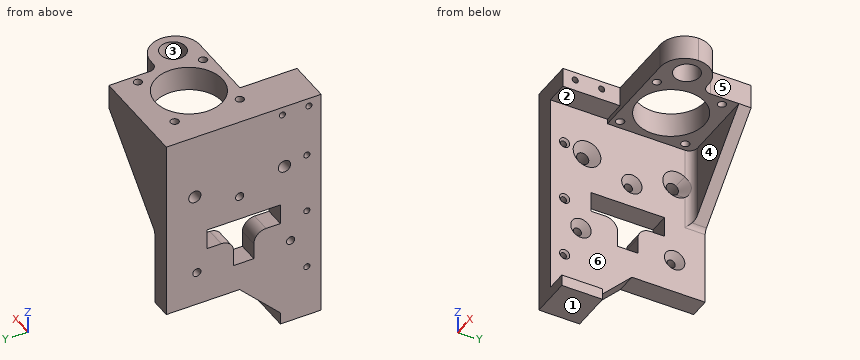
Autodesk Inventor part; units mm, degrees
ref_plane "YZ Plane" through (0, 0, 0) normal (1, 0, 0) x (0, 1, 0)
ref_plane "XZ Plane" through (0, 0, 0) normal (0, 1, 0) x (-1, 0, 0)
ref_plane "XY Plane" through (0, 0, 0) normal (0, 0, 1) x (1, 0, 0)
sketch "Sketch1" plane through (0, 0, 0) normal (1, 0, 0) x (0, 1, 0)
  line L0 (-23.3447, 18.3788) -> (14.6553, 18.3788)
  line L1 (14.6553, 18.3788) -> (14.6553, -36.6212)
  line L2 (14.6553, -36.6212) -> (-23.3447, -36.6212)
  line L3 (-23.3447, -36.6212) -> (-23.3447, 18.3788)
  point P0 (0, 0)
  dimension "d0" = 38
  dimension "d1" = 55
extrude "Extrusion1" add sketch "Sketch1" along normal blind 5
sketch "Sketch2" plane through (5, 0, 0) normal (1, 0, 0) x (0, 0, -1)
  line L0 (36.6212, 14.6553) -> (-18.3788, 14.6553)
  line L1 (-18.3788, 14.6553) -> (-12.3788, 14.6553)
  line L2 (-12.3788, 14.6553) -> (-12.3788, -9.3447)
  line L3 (-12.3788, -9.3447) -> (-18.3788, -9.3447)
  line L4 (-18.3788, -9.3447) -> (-18.3788, 14.6553)
  point P0 (0, 0)
  dimension "d4" = 24
  dimension "d5" = 6
extrude "Extrusion2" add sketch "Sketch2" along normal blind 20
sketch "Sketch3" plane through (5, -9.3447, 12.3788) normal (0, 0, -1) x (-1, 0, 0)
  circle A0 centre (-10, 10) radius 8.25
  line L0 (-20, 0) -> (-20, 24)
  line L1 (0, 0) -> (-20, 0)
  circle A1 centre (-18, 2) radius 1
  circle A2 centre (-18, 18) radius 1
  circle A3 centre (-2, 2) radius 1
  circle A4 centre (-2, 18) radius 1
  point P0 (5, 9.3447)
  dimension "d8" = 16.5
  dimension "d9" = 10
  dimension "d10" = 10
  dimension "d11" = 2
  dimension "d12" = 2
  dimension "d13" = 2
  dimension "d14" = 2
  dimension "d15" = 8
  dimension "d16" = 8
  dimension "d17" = 8
  dimension "d18" = 8
  dimension "d19" = 8
  dimension "d20" = 8
  dimension "d21" = 8
  dimension "d22" = 8
extrude "Extrusion3" cut sketch "Sketch3" against normal through all
sketch "Sketch4" plane through (5, -9.3447, 12.3788) normal (0, 0, -1) x (-1, 0, 0)
  line L0 (-20, 24) -> (-20, 0)
  line L1 (0, 24) -> (0, 0)
  line L2 (-20, 24) -> (0, 24)
  line L3 (0, 24) -> (0, 21)
  line L4 (0, 21) -> (-20, 21)
  line L5 (-20, 21) -> (-20, 24)
  point P0 (5, 9.3447)
  dimension "d25" = 3
extrude "Extrusion4" add sketch "Sketch4" along normal blind 20
sketch "Sketch5" plane through (5, 11.6553, 12.3788) normal (0, -1, 0) x (1, 0, 0)
  line L0 (0, -20) -> (0, 0)
  line L1 (20, 6) -> (20, 0)
  line L2 (0, -20) -> (20, 0)
  line L3 (20, 0) -> (20, -20)
  line L4 (20, -20) -> (0, -20)
  line L5 (20, -20) -> (0, -20)
  point P0 (-5, -12.3788)
extrude "Extrusion5" cut sketch "Sketch5" against normal through all
fillet "Fillet1" radius 2 2 edges at (5, 11.6553, 2.3788) (5, 13.1553, -7.6212)
sketch "Sketch6" plane through (5, 0, 0) normal (1, 0, 0) x (0, 0, -1)
  circle A0 centre (1.6212, -3.3447) radius 1
  line L0 (36.6212, 14.6553) -> (8.4496, 14.6553)
  line L1 (36.6212, -23.3447) -> (36.6212, 14.6553)
  point P0 (0, 0)
  dimension "d31" = 2
  dimension "d32" = 18
  dimension "d33" = 35
extrude "Extrusion6" cut sketch "Sketch6" against normal through all
sketch "Sketch7" plane through (5, 0, 0) normal (1, 0, 0) x (0, 0, -1)
  circle A0 centre (-2.3788, -14.3447) radius 1.5
  circle A1 centre (-2.3788, 7.6553) radius 1.5
  circle A2 centre (1.6212, -3.3447) radius 1
  point P0 (0, 0)
  dimension "d36" = 3
  dimension "d37" = 3
  dimension "d38" = 4
  dimension "d39" = 11
  dimension "d40" = 11
  dimension "d41" = 4
extrude "Extrusion7" cut sketch "Sketch7" against normal through all contours A0 | A1
chamfer "Chamfer1" distance 1.5 angle 45 1 edges at (5, -3.3447, -0.6212)
chamfer "Chamfer2" distance 1.9 angle 45 2 edges at (5, -14.3447, 3.8788) (5, 7.6553, 3.8788)
sketch "Sketch8" plane through (5, 0, 0) normal (1, 0, 0) x (0, 0, -1)
  line L0 (36.6212, 14.6553) -> (-18.3788, 14.6553)
  line L1 (36.6212, 14.6553) -> (26.6212, 14.6553)
  line L2 (26.6212, 14.6553) -> (26.6212, -13.3447)
  line L3 (26.6212, -13.3447) -> (36.6212, -13.3447)
  line L4 (36.6212, -13.3447) -> (36.6212, 14.6553)
  point P0 (0, 0)
  dimension "d50" = 28
  dimension "d51" = 10
extrude "Extrusion8" cut sketch "Sketch8" against normal through all
chamfer "Chamfer3" distance 10 angle 45 1 edges at (2.5, -13.3447, -26.6212)
sketch "Sketch9" plane through (5, 0, 0) normal (1, 0, 0) x (0, 0, -1)
  circle A0 centre (18.1212, -15.8447) radius 1
  circle A1 centre (18.1212, 7.1553) radius 1
  line L0 (26.6212, 14.6553) -> (8.4496, 14.6553)
  line L1 (36.6212, -23.3447) -> (36.6212, -13.3447)
  line L2 (-18.3788, -23.3447) -> (36.6212, -23.3447)
  point P0 (0, 0)
  dimension "d57" = 2
  dimension "d58" = 2
  dimension "d59" = 7.5
  dimension "d60" = 18.5
  dimension "d61" = 7.5
  dimension "d62" = 18.5
extrude "Extrusion9" cut sketch "Sketch9" against normal through all
chamfer "Chamfer4" distance 1.5 angle 45 2 edges at (5, -15.8447, -17.1212) (5, 7.1553, -17.1212)
sketch "Sketch10" plane through (5, 0, 0) normal (1, 0, 0) x (0, 0, -1)
  circle A0 centre (26.6212, -19.8447) radius 0.75
  circle A1 centre (11.6212, -19.8447) radius 0.75
  circle A2 centre (-3.3788, -19.8447) radius 0.75
  line L0 (-18.3788, -23.3447) -> (36.6212, -23.3447)
  line L1 (36.6212, -23.3447) -> (36.6212, -13.3447)
  line L2 (-18.3788, -9.3447) -> (-18.3788, -23.3447)
  point P0 (0, 0)
  dimension "d68" = 1.5
  dimension "d69" = 1.5
  dimension "d70" = 1.5
  dimension "d71" = 3.5
  dimension "d72" = 10
  dimension "d73" = 3.5
  dimension "d74" = 15
  dimension "d76" = 3.5
  dimension "d95" = 15
extrude "Extrusion10" cut sketch "Sketch10" against normal through all
sketch "Sketch15" plane through (5, 0, 0) normal (1, 0, 0) x (0, 0, -1)
  line L0 (36.6212, -23.3447) -> (36.6212, -13.3447)
  line L1 (36.6212, -23.3447) -> (39.6212, -23.3447)
  line L2 (39.6212, -23.3447) -> (39.6212, -13.3447)
  line L3 (39.6212, -13.3447) -> (36.6212, -13.3447)
  line L4 (36.6212, -13.3447) -> (36.6212, -23.3447)
  point P0 (0, 0)
  dimension "d96" = 3
  dimension "d97" = 10
extrude "Extrusion15" add sketch "Sketch15" against normal up to surface (5 mm away)
sketch "Sketch16" plane through (5, 0, 0) normal (1, 0, 0) x (0, 0, -1)
  line L0 (-18.3788, -23.3447) -> (39.6212, -23.3447)
  line L1 (39.6212, -13.3447) -> (36.6212, -13.3447)
  line L2 (39.6212, -23.3447) -> (36.8212, -23.3447)
  line L3 (36.8212, -23.3447) -> (36.8212, -13.3447)
  line L4 (36.8212, -13.3447) -> (39.6212, -13.3447)
  line L5 (39.6212, -13.3447) -> (39.6212, -23.3447)
  point P0 (0, 0)
  dimension "d100" = 2.8
extrude "Extrusion16" add sketch "Sketch16" along normal blind 5
sketch "Sketch17" plane through (5, 0, 0) normal (1, 0, 0) x (0, 0, -1)
  line L0 (-18.3788, -23.3447) -> (39.6212, -23.3447)
  line L1 (-12.3788, -9.3447) -> (-18.3788, -9.3447)
  line L2 (-18.3788, -23.3447) -> (-13.5788, -23.3447)
  line L3 (-13.5788, -23.3447) -> (-13.5788, -9.3447)
  line L4 (-13.5788, -9.3447) -> (-18.3788, -9.3447)
  line L5 (-18.3788, -9.3447) -> (-18.3788, -23.3447)
  point P0 (0, 0)
  dimension "d103" = 4.8
extrude "Extrusion17" add sketch "Sketch17" along normal blind 5.5
sketch "Sketch18" plane through (10.5, 0, 0) normal (1, 0, 0) x (0, 0, -1)
  circle A0 centre (-16.3788, -20.3447) radius 0.75
  circle A1 centre (-16.3788, -13.8447) radius 0.75
  line L0 (-18.3788, -23.3447) -> (-13.5788, -23.3447)
  line L1 (-18.3788, -9.3447) -> (-18.3788, -23.3447)
  point P0 (0, 0)
  point P1 (-15.9788, -23.3447)
  dimension "d106" = 1.5
  dimension "d107" = 1.5
  dimension "d108" = 6.5
  dimension "d109" = 3
  dimension "d110" = 2
  dimension "d111" = 2
extrude "Extrusion18" cut sketch "Sketch18" against normal through all
sketch "Sketch19" plane through (5, 0, 0) normal (1, 0, 0) x (0, 0, -1)
  line L0 (7.6212, -13.3447) -> (12.6212, -13.3447)
  line L1 (12.6212, -13.3447) -> (12.6212, 4.6553)
  line L2 (12.6212, 4.6553) -> (7.6212, 4.6553)
  line L3 (7.6212, 4.6553) -> (7.6212, -13.3447)
  line L4 (26.6212, 14.6553) -> (8.4496, 14.6553)
  line L5 (-13.5788, -23.3447) -> (36.8212, -23.3447)
  line L6 (26.6212, -3.3447) -> (26.6212, 14.6553)
  point P0 (0, 0)
  dimension "d114" = 5
  dimension "d115" = 10
  dimension "d116" = 10
  dimension "d117" = 14
extrude "Extrusion19" cut sketch "Sketch19" against normal through all
chamfer "Chamfer5" distance 0.5 angle 45 3 edges at (5, -19.8447, 4.1288) (5, -19.8447, -10.8712) (5, -19.8447, -25.8712)
sketch "Sketch20" plane through (25, 0, 0) normal (1, 0, 0) x (0, 0, -1)
  line L0 (-12.3788, -9.3447) -> (-13.5788, -9.3447)
  line L1 (-18.3788, 14.6553) -> (-18.3788, -9.3447)
  line L2 (-12.3788, -9.3447) -> (-18.3788, -9.3447)
  line L3 (-18.3788, -9.3447) -> (-18.3788, 2.6553)
  line L4 (-18.3788, 2.6553) -> (-12.3788, 2.6553)
  line L5 (-12.3788, 2.6553) -> (-12.3788, -9.3447)
  point P0 (0, 0)
  dimension "d123" = 12
extrude "Extrusion20" add sketch "Sketch20" along normal blind 9
sketch "Sketch21" plane through (0, -23.3447, 18.3788) normal (0, 0, 1) x (1, 0, 0)
  circle A0 centre (29, 20) radius 3.1
  line L0 (25, 26) -> (34, 26)
  line L1 (34, 26) -> (34, 14)
  point P0 (0, 23.3447)
  dimension "d126" = 6.2
  dimension "d127" = 6
  dimension "d128" = 5
extrude "Extrusion21" cut sketch "Sketch21" against normal through all
fillet "Fillet3" radius 6 2 edges at (34, -9.3447, 15.3788) (34, 2.6553, 15.3788)
sketch "Sketch22" plane through (5, 0, 0) normal (1, 0, 0) x (0, 0, -1)
  line L0 (12.6212, -13.3447) -> (12.6212, 4.6553)
  line L1 (12.6212, -6.8447) -> (19.6212, -6.8447)
  line L2 (19.6212, -6.8447) -> (19.6212, -1.8447)
  line L3 (19.6212, -1.8447) -> (12.6212, -1.8447)
  line L4 (12.6212, -1.8447) -> (12.6212, -6.8447)
  line L5 (7.6212, 4.6553) -> (12.6212, 4.6553)
  point P0 (0, 0)
  dimension "d134" = 5
  dimension "d135" = 6.5
  dimension "d136" = 7
extrude "Extrusion22" cut sketch "Sketch22" against normal through all
fillet "Fillet5" radius 3 2 edges at (2.5, -6.8447, -12.6212) (2.5, -1.8447, -12.6212)
fillet "Fillet6" radius 2 1 edges at (25, 2.6553, 15.3788)
properties part number "Z_motor_holder" material "ABS Plastic"
Part model, mm, in its own coordinate system. Face numbers are marked on the shaded views. A direction names the side the tool comes from. Give positions to 0.01 mm unless a question says otherwise; leave off trailing zeros. Order: outer loops, then holes, each group sorted by start corner. A loop starts at its lowest first (then second) coordinate and runs counter-clockwise, first axis right, second up. Notation, with made-up numbers: (-26, 52) - (-11, 52) arc R18 cw to (-11, 57) - close; hole circle Ø9 at (-20.75, 89). An arc over 180 degrees is marked (long way). One line per question, with ' | ' between items.
1. Which spindle directions (+Z, -Z, +X, -X, +Y, -Y) get a long thin tool onto all of the face, cutting with end or side? Do the marked faces 4, 5 and 6. Say none if no direction does.
Filled in:
face 4: -Z, +X, -Y | face 5: +Z, -Z, +X, +Y | face 6: +X, -Y
2. Drill centre lines: probe 1 along Y at (x, z) = (14.5, 15); probe 2 along Y at (x, z) = (18, 8); probe 3 along Z at (x, y) = (4, -6). Where is each one in solid material? Low to high.
Filled in:
probe 1: -9.34 to -7.58, 8.89 to 14.66 | probe 2: 11.66 to 14.66 | probe 3: -29.28 to -19.62, -7.62 to 18.38
3. Band-saw the part on A-A on x = 15. List the corners of the cut face in (y, z).
Filled in:
outline: (-9.34, 12.38) - (-7.59, 12.38) - (-7.59, 18.38) - (-9.34, 18.38) - close; (8.91, 12.38) - (11.66, 12.38) - (11.66, 2.38) - (14.66, 2.38) - (14.66, 18.38) - (8.91, 18.38) - close
4. Drop flat-ended pins along their axis: P1, Ø0.8, axis at y = -17, z = -38, coming from the +X side; P2, Ø5.5, axis at x = 3, y = 6.5, coming from the -Z side; P3, Ø12, axis at x = 6, z = -28, coming from the +Y side; P4, Ø5.5, axis at y = -15, z = 17, coming from the +X side. Give the stop position or say it passes through.
Filled in:
P1: x = 10 | P2: z = -26.62 | P3: y = 14.66 | P4: x = 10.5
5. Band-saw the part on C-C on z = -30.5. List the corners of the cut face in (x, y), then the cut area to 3 significant figures.
Filled in:
outline: (0, -23.34) - (5, -23.34) - (5, -7.22) - (0, -7.22) - close | area: 80.6 mm²
6. Pull direction Z, two halves, no side cores. Call the marked faces 1, 2 and 3: +Z half, -Z half, draft (parallel to the pull), parting line (faces both ways), or undercut.
Filled in:
face 1: -Z half | face 2: undercut | face 3: draft
7. Band-saw the part on B-B on x = 30. List the corners of the cut face in (y, z), then the cut area to 3 significant figures.
Filled in:
outline: (-9, 12.38) - (-6.28, 12.38) - (-6.28, 18.38) - (-9, 18.38) - close; (-0.41, 12.38) - (2.31, 12.38) - (2.31, 18.38) - (-0.41, 18.38) - close | area: 32.7 mm²
